Autodesk Inventor part; units mm, degrees
ref_plane "YZ Plane" through (0, 0, 0) normal (1, 0, 0) x (0, 1, 0)
ref_plane "XZ Plane" through (0, 0, 0) normal (0, 1, 0) x (-1, 0, 0)
ref_plane "XY Plane" through (0, 0, 0) normal (0, 0, 1) x (1, 0, 0)
sketch "Sketch1" plane through (0, 0, 0) normal (0, 0, 1) x (1, 0, 0)
  circle A0 centre (0, 0) radius 40
  dimension "d0" = 80
extrude "Extrusion1" add sketch "Sketch1" along normal blind 3
sketch "Sketch2" plane through (0, 0, 3) normal (0, 0, 1) x (1, 0, 0)
  circle A0 centre (0, 0) radius 10
  dimension "d3" = 20
extrude "Extrusion2" add sketch "Sketch2" against normal blind 160
sketch "Sketch3" plane through (0, 0, 0) normal (1, 0, 0) x (0, 1, 0)
  circle A0 centre (-59.9652, -126.9652) radius 30.0348
  line L0 (-10, -157) -> (10, -157)
  line L1 (0, -157) -> (0, -174.595) construction
  line L2 (-90, -126.9652) -> (-90, -88.517)
  line L3 (-59.9652, -126.9652) -> (0, -126.9652) construction
  line L4 (0, -126.9652) -> (0, -131.9652)
  line L5 (0, -131.9652) -> (-30.3494, -131.9652)
  line L6 (0, -126.9652) -> (0, -121.9652)
  line L7 (0, -121.9652) -> (-30.3494, -121.9652)
  point P0 (0, 0)
  dimension "d8" = 90
  dimension "d9" = 5
  dimension "d10" = 5
extrude "Extrusion3" add sketch "Sketch3" along normal mid plane 4
sketch "Sketch4" plane through (0, 0, -157) normal (0, 0, -1) x (-1, 0, 0)
  circle A0 centre (-13.7706, 13.7706) radius 35.6894
  point P0 (0, 0)
extrude "Extrusion4" cut sketch "Sketch4" against normal up to surface (25.0348 mm away)
pattern_circular "Circular Pattern1" count 3 over 360 about axis through (0, 0, 3) along (0, 0, -1) of "Extrusion3"
properties part number "manometro idealmente"
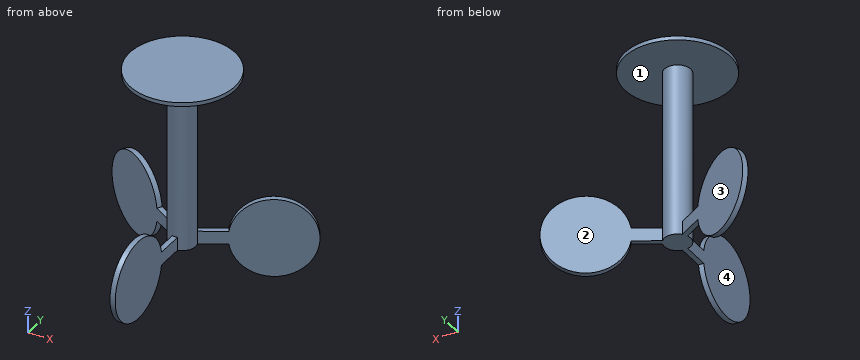
Model file for the job. Use its own axes, mm. Face numbers are marked on the shaded views. Give positions to 0.01 mm unless a question says otherwise; leave off trailing zeros. Loops run counter-clockwise (first coordinate to the right, second up) from the corner with the lowest first, then second, coordinate; pieces in that order, holes last.
Item 1: Mould opens along X. For the marked faces 1, 2, 3 and 4 say: +X half, -X half, draft (parallel to the pull), parting line (faces both ways), or undercut.
Check values:
face 1: draft
face 2: undercut
face 3: undercut
face 4: -X half
Item 2: Slice it at C-C (z = -56.5). Write the cut outline in (x, y).
Check values:
outline: circle Ø20 at (0, 0)
Item 3: Slice it at D-D (y = -52). Write the cut outline in (x, z).
Check values:
outline: (-2, -155.92) - (2, -155.92) - (2, -98.01) - (-2, -98.01) - close
Item 4: Slice it at B-B (z = -135.5). Write the cut outline in (x, y), plus the area to 3 significant figures.
Check values:
outline: (-77.87, 42.65) - (-27.99, 13.85) - (-25.99, 17.32) - (-75.87, 46.11) - close; (-2, -88.76) - (2, -88.76) - (2, -31.17) - (-2, -31.17) - close; (25.99, 17.32) - (27.99, 13.85) - (77.87, 42.65) - (75.87, 46.11) - close
area: 691 mm2
Item 5: Drop flat-ended pins along their axis: P1, Ø14, axis at x = -7.5, y = 2.5, coming from the -Z side; P2, Ø1.5, axis at y = -0.5, z = -106, coming from the +X side; P3, Ø1.5, axis at y = -20, z = -129, coming from the -X side. Give the stop position or say it passes through.
Check values:
P1: stops at z = -131.97
P2: stops at x = 10
P3: stops at x = -2
Item 6: Drill centre lines: line 1 along X through (y, z) = (-27, -123); line 2 along X through (y, z) = (-1, -58); line 3 along Z through (x, y) = (-3, 13.5). Where is each one in solid material? Low to high.
Check values:
line 1: x = -2 to 2
line 2: x = -9.95 to 9.95
line 3: z = 0 to 3
Item 7: Slice it at A-A (y = 0). Write the cut outline in (x, z), plus the area to 3 significant figures.
Check values:
outline: (-40, 0) - (-10, 0) - (-10, -131.97) - (10, -131.97) - (10, 0) - (40, 0) - (40, 3) - (-40, 3) - close
area: 2,880 mm2
